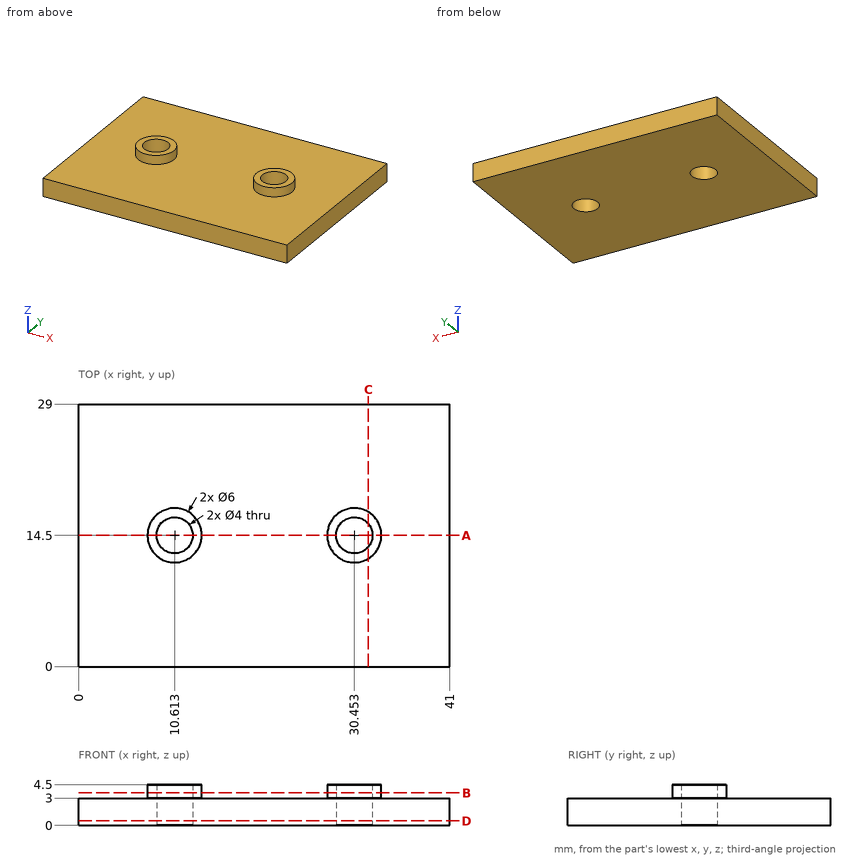
Part print with two shaded views. Sizes in mm from the minimum x, y, z corner. Give positions to 0.01 mm unless a question says otherwise; leave off trailing zeros. Order: outer loops, then holes, each group sorted by start corner. A loop starts at its lowest first (then second) coordinate and runs counter-clockwise, first axis right, second up. Notation, with made-up numbers: M 19.25,81.25 L 32.25,81.25 A23 ccw 32.25,109.25 Z; hole C 28.5,52 d4. An arc over 180 degrees is marked long. Write item = value, one per line.
Q1. Cut at A-A, the plane y = 14.5. List the corners of the cut face in (x, z), then the cut area to 3 significant figures.
Derived:
outline = M 0,0 L 8.61,0 L 8.61,4.5 L 7.61,4.5 L 7.61,3 L 0,3 Z; M 12.61,0 L 28.45,0 L 28.45,4.5 L 27.45,4.5 L 27.45,3 L 13.61,3 L 13.61,4.5 L 12.61,4.5 Z; M 32.45,0 L 41,0 L 41,3 L 33.45,3 L 33.45,4.5 L 32.45,4.5 Z
area = 105 mm2
Q2. Cut at D-D, the plane z = 0.5. List the corners of the cut face in (x, y), then the cut area to 3 significant figures.
Derived:
outline = M 0,0 L 41,0 L 41,29 L 0,29 Z; hole C 10.61,14.5 d4; hole C 30.45,14.5 d4
area = 1,160 mm2
Q3. Cut at C-C, the plane x = 32. List the corners of the cut face in (y, z), then the cut area to 3 significant figures.
Derived:
outline = M 0,0 L 13.23,0 L 13.23,4.5 L 11.93,4.5 L 11.93,3 L 0,3 Z; M 15.77,0 L 29,0 L 29,3 L 17.07,3 L 17.07,4.5 L 15.77,4.5 Z
area = 83.3 mm2
Q4. Flat gauge pins, fed straight in: pin 1 (3.5 mm diameter, centred on x = 10.61, y = 14.5, fed in from -Z); pin 2 (4 mm diameter, centred on x = 18, y = 11.5, fed in from +Z). Where does each tip first touch, or does it go through?
Derived:
pin_1 = through
pin_2 = 3
Q5. Drill centre lines: line 1 (Z direction, x = 37.5, y = 17); line 2 (Y direction, x = 11.5, z = 3.4) (1 decimal); line 3 (X direction, y = 12.25, z = 3.2). Where is each one in solid material? Low to high. Write a range as [from, to].
Derived:
line_1 = [0, 3]
line_2 = [11.6, 12.7], [16.3, 17.4]
line_3 = [8.63, 12.6], [28.47, 32.44]
Q6. Cut at B-B, the plane z = 3.6. List the corners of the cut face in (x, y).
Derived:
outline = C 10.61,14.5 d6; C 30.45,14.5 d6; hole C 10.61,14.5 d4; hole C 30.45,14.5 d4
